```python
from build123d import *

# Parameters (mm, degrees)
SKETCH1_R           = 15
BOSS_EXTRUDE1_DEPTH = 60
SKETCH2_R           = 7.5
CUT_EXTRUDE1_DEPTH  = 125.233650836
SKETCH3_W           = 15
SKETCH3_H           = 32
CUT_EXTRUDE2_DEPTH  = 114.176852757
RIB3_REACH          = 127.734
SKETCH4_WALL_W      = 331.787548758
SKETCH4_WALL_H      = 10


with BuildPart() as part:
    # Sketch1 → Boss-Extrude1 (new body)
    with BuildSketch(Plane.XY):
        with BuildLine():
            Line((-12, 52), (12, 52))
            Line((12, 52), (20, 0))
            Line((20, 0), (33, 0))
            Line((33, 0), (33, 5))
            Line((33, 5), (53, 5))
            Line((53, 5), (53, 15))
            Line((53, 15), (30, 15))
            Line((30, 15), (30, 80))
            ThreePointArc((30, 80), (0, 110), (-30, 80))
            Line((-30, 80), (-30, 15))
            Line((-30, 15), (-53, 15))
            Line((-53, 15), (-53, 5))
            Line((-53, 5), (-33, 5))
            Line((-33, 5), (-33, 0))
            Line((-33, 0), (-20, 0))
            Line((-20, 0), (-12, 52))
        make_face()
        with Locations((0, 80)):
            Circle(SKETCH1_R, mode=Mode.SUBTRACT)
    extrude(amount=BOSS_EXTRUDE1_DEPTH)

    # Sketch2 → Cut-Extrude1 (cut, through all)
    with BuildSketch(Plane(origin=(0, 15, 0), x_dir=(1, 0, 0), z_dir=(0, 1, 0))):
        with Locations(Location((-41.5, -12.5, 0), (0, 0, 180))):
            Circle(SKETCH2_R)
        with Locations(Location((-41.5, -47.5, 0), (0, 0, 180))):
            Circle(SKETCH2_R)
        with Locations(Location((41.5, -47.5, 0), (0, 0, 270))):
            Circle(SKETCH2_R)
        with Locations(Location((41.5, -12.5, 0), (0, 0, 270))):
            Circle(SKETCH2_R)
    extrude(amount=-CUT_EXTRUDE1_DEPTH, mode=Mode.SUBTRACT)

    # Sketch3 → Cut-Extrude2 (cut, through all)
    with BuildSketch(Plane(origin=(0, 80, 0), x_dir=(1, 0, 0), z_dir=(0, 1, 0))):
        with Locations((0, -30)):
            Rectangle(SKETCH3_W, SKETCH3_H)
    extrude(amount=CUT_EXTRUDE2_DEPTH, mode=Mode.SUBTRACT)

    # Sketch4 wall → Rib3 (add, up to next)
    with BuildSketch(Plane(origin=(40.746781429, 52.193529473, 30), x_dir=(0.312901964861, -0.949785428603, 0), z_dir=(0.949785428603, 0.312901964861, 0)), mode=Mode.PRIVATE) as rib3_sk1:
        Rectangle(SKETCH4_WALL_W, SKETCH4_WALL_H)
    rib3_tool1 = extrude(rib3_sk1.sketch, amount=-RIB3_REACH, mode=Mode.PRIVATE) - part.part
    rib3 = rib3_tool1.solids().sort_by_distance((40.746781429, 52.193529473, 30))[0]
    add(rib3)

    # Mirror1: Rib3 across plane
    add(rib3.mirror(Plane(origin=(0, 0, 0), x_dir=(0, 0, 1), z_dir=(1, 0, 0))))


solid = part.part
```
Geometry: final body of the model. Coordinates: model frame, mm. A direction names the side the tool comes from. Round coordinates to 2 decimals unless told otherwise and drop trailing zeros. Write each loop counter-clockwise with the first axis right and the second up, starting at its lowest first coordinate (ties: lowest second). Pieces come first, ordered by that corner, then holes. Notation, with made-up numbers: M -28,36.25 L -11,36.25 A29 ccw -11,69.25 Z; hole C -28,54.25 d6. An arc over 180 degrees is marked long. Answer in a Markdown table with one row per item. Add a question column.
(1) Cut plane C-C, the plane y = 73.5. Return the cut outline in (x, z), then the cut area to 3 significant figures.
(2) Cut plane D-D, the plane z = 9.5. Return the cut outline in (x, y).
(3) Reachability of faces 4 (the face through (0, 52, 30)), 5 (the face through (0, 101, 46)), 6 (the face through (-36, 15, 7)), 7 (the face through (-36, 15, 42)), 8 (the face through (30, 47, 47)) from +Z, -Z, +X, -X, +Y, -Y: full face, straight path, thin tool, end or side. Return the list, or none.
(4) Ray query, L1, parallel to X at y = 7, z = 12; L2, parallel to Y at x = -39, z = 39.5; L3, parallel to Y at x = -11, z = 39. Return the intervals inside material, ascending.
(5) Cut plane B-B, the plane x = 0. Return the cut outline in (y, z), then the cut area to 3 significant figures.
(6) Contact query for flat-ended pins moving along their axis: pin 1 (12.5 mm diameter, centred on x = -40.5, y = 39.5, fed in from +Z); pin 2 (12 mm diameter, centred on y = 55.5, z = 43.5, fed in from +X); pin 3 (9 mm diameter, centred on x = 41.5, z = 47.5, fed in from +Y); pin 4 (19 mm diameter, centred on x = -0.5, z = 24, fed in from -Y). Output: stop coordinate, or through.
(7) Cut plane A-A, the plane z = 47.5. Return the cut outline in (x, y).
(8) Draft query along X for faces 1 (the face through (10.878, 107.958, 29.58)), 2 (the face through (-3.252, 65.357, 29.58)), 3 (the face through (47, 15, 7)). Return one class per face: pulls with the +X half, pulls with the -X half, needs draft (parallel to the pull), parting line crosses it, or undercut.
Established:
| question | item | result |
|---|---|---|
| 1 | outline | M -33.73,25 L -30,25 L -30,0 L -13.52,0 L -13.52,60 L -30,60 L -30,35 L -33.73,35 Z; M 13.52,0 L 30,0 L 30,25 L 33.73,25 L 33.73,35 L 30,35 L 30,60 L 13.52,60 Z |
| 1 | area | 2,050 mm² |
| 2 | outline | M -53,5 L -48.37,5 L -48.37,15 L -53,15 Z; M -34.63,5 L -33,5 L -33,0 L -20,0 L -12,52 L 12,52 L 20,0 L 33,0 L 33,5 L 34.63,5 L 34.63,15 L 30,15 L 30,80 A30 ccw -30,80 L -30,15 L -34.63,15 Z; M 48.37,5 L 53,5 L 53,15 L 48.37,15 Z; hole C 0,80 d30 |
| 3 | face 4 | +Z, -Z, -Y |
| 3 | face 5 | +Y |
| 3 | face 6 | -Z, -X, +Y |
| 3 | face 7 | +Z, -X, +Y |
| 3 | face 8 | +Z, +X, +Y |
| 4 | L1 | -53 to -48.98, -34.02 to -18.92, 18.92 to 34.02, 48.98 to 53 |
| 4 | L2 | 5 to 15 |
| 4 | L3 | 52 to 69.8, 90.2 to 107.91 |
| 5 | outline | M 52,0 L 65,0 L 65,60 L 52,60 Z; M 95,0 L 110,0 L 110,14 L 95,14 Z; M 95,46 L 110,46 L 110,60 L 95,60 Z |
| 5 | area | 1,200 mm² |
| 6 | pin 1 | z = 35 |
| 6 | pin 2 | x = 30 |
| 6 | pin 3 | through |
| 6 | pin 4 | y = 52 |
| 7 | outline | M -53,5 L -49,5 L -49,15 L -53,15 Z; M -34,5 L -33,5 L -33,0 L -20,0 L -12,52 L 12,52 L 20,0 L 33,0 L 33,5 L 34,5 L 34,15 L 30,15 L 30,80 A30 ccw -30,80 L -30,15 L -34,15 Z; M 49,5 L 53,5 L 53,15 L 49,15 Z; hole C 0,80 d30 |
| 8 | face 1 | parting line crosses it |
| 8 | face 2 | undercut |
| 8 | face 3 | needs draft |
